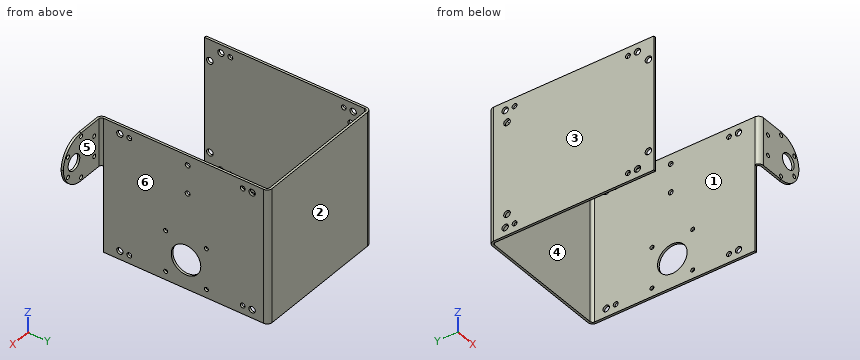
from build123d import *

# Parameters (mm, degrees)
F1_DEPTH  = 101.8535682
F2_R      = 1.5
F2_R_2    = 5.969
F3_DEPTH  = 1.70942
F4_R      = 1.98374
F5_R      = 3.69316
F6_R      = 2.4125047
F6_R_2    = 1.8288
F7_DEPTH  = 105.01884
F8_R      = 11.2530001
F8_R_2    = 1.5
F8_R_3    = 1.8288
F9_DEPTH  = 103.30942
F10_W     = 3.69316
F10_H     = 65.5315682
F11_DEPTH = 40.01516
F12_R     = 18.16099
F13_R     = 2.5
F14_DEPTH = 1.70942


# Not quite as in the source:
# - a fillet or chamfer is up to 0.001 mm smaller than in the source, because OpenCascade refuses the exact size
# - a feature names something its author has since deleted; it is built from what else it names


with BuildPart() as f1:
    # F0 (on Top) → F1 (new body)
    with BuildSketch(Plane.XY):
        Polygon((-1.70942, 0), (0, 0), (0, 123.945777), (101.6, 123.945777), (101.6, -3.69316), (141.61516, -3.69316), (141.61516, -1.98374), (103.30942, -1.98374), (103.30942, 125.655197), (-1.70942, 125.655197), align=None)
    extrude(amount=F1_DEPTH)

    # F2 (on face) → F3 (cut, through all)
    with BuildSketch(Plane.XZ.offset(3.69316)):
        with Locations((136.8723576062, 91.4395682)):
            Circle(F2_R)
        with Locations((130.82016, 83.6925682)):
            Circle(F2_R_2)
        with Locations((136.8723576062, 75.9455682)):
            Circle(F2_R)
        with Locations((123.45416, 99.1865682)):
            Circle(F2_R)
        with Locations((110.0359623938, 91.4395682)):
            Circle(F2_R)
        with Locations((110.0359623938, 75.9455682)):
            Circle(F2_R)
        with Locations((123.45416, 68.1985682)):
            Circle(F2_R)
    extrude(amount=-F3_DEPTH, mode=Mode.SUBTRACT)

    # F4
    f4_edges = [f1.edges().sort_by_distance(p)[0] for p in [
        (0, 123.945777, 50.926784),
        (101.6, 123.945777, 50.926784),
        (103.30942, -1.98374, 50.926784),
    ]]
    fillet(f4_edges, radius=F4_R)

    # F5
    f5_edges = [f1.edges().sort_by_distance(p)[0] for p in [
        (-1.70942, 125.655197, 50.926784),
        (103.30942, 125.655197, 50.926784),
        (101.6, -3.69316, 50.926784),
    ]]
    fillet(f5_edges, radius=F5_R)

    # F6 (on face) → F7 (cut, through all)
    with BuildSketch(Plane(origin=(-1.70942, 0, 0), x_dir=(0, -1, 0), z_dir=(-1, 0, 0))):
        with Locations((-12.5063584, 95.4723182)):
            Circle(F6_R)
        with Locations((-19.6813584, 95.4723182)):
            Circle(F6_R_2)
        with Locations((-105.9738466, 95.4723182)):
            Circle(F6_R_2)
        with Locations((-105.9738466, 6.38125)):
            Circle(F6_R_2)
        with Locations((-19.6813584, 6.38125)):
            Circle(F6_R_2)
        with Locations((-113.1488466, 95.4723182)):
            Circle(F6_R)
        with Locations((-113.1488466, 6.38125)):
            Circle(F6_R)
        with Locations((-12.5063584, 6.38125)):
            Circle(F6_R)
    extrude(amount=-F7_DEPTH, mode=Mode.SUBTRACT)

    # F8 (on face) → F9 (cut, through all)
    with BuildSketch(Plane.YZ.offset(103.30942)):
        with Locations((62.8276025004, 21.8812444)):
            Circle(F8_R)
        with Locations((47.3276081004, 37.3812388)):
            Circle(F8_R_2)
        with Locations((78.3275969004, 37.3812388)):
            Circle(F8_R_2)
        with Locations((78.3275969004, 6.38125)):
            Circle(F8_R_2)
        with Locations((47.3276081004, 6.38125)):
            Circle(F8_R_2)
        with Locations((64.05626, 72.9453964)):
            Circle(F8_R_3)
        with Locations((64.05626, 94.43974)):
            Circle(F8_R_3)
    extrude(amount=-F9_DEPTH, mode=Mode.SUBTRACT)

    # F10 (on face) → F11 (cut, through all)
    with BuildSketch(Plane.YZ.offset(141.61516)):
        with Locations((-1.84658, 32.7657841)):
            Rectangle(F10_W, F10_H)
    extrude(amount=-F11_DEPTH, mode=Mode.SUBTRACT)

    # F12 (radius 18.161 in the source; OpenCascade refuses exactly that, so slightly less here)
    f12_edges = [f1.edges().sort_by_distance(p)[0] for p in [
        (141.61516, -2.83845, 65.531568),
        (141.61516, -2.83845, 101.853568),
    ]]
    fillet(f12_edges, radius=F12_R)

    # F13 (on face) → F14 (cut, through all)
    with BuildSketch(Plane(origin=(-1.70942, 0, 0), x_dir=(0, -1, 0), z_dir=(-1, 0, 0))):
        with Locations((-111.7494286, 16.056229)):
            Circle(F13_R)
        with Locations((-4.0875, 16.056229)):
            Circle(F13_R)
        with Locations((-4.0875, 85.7973392)):
            Circle(F13_R)
        with Locations((-111.7494286, 85.7973392)):
            Circle(F13_R)
    extrude(amount=-F14_DEPTH, mode=Mode.SUBTRACT)


solid = f1.part
Part model, mm, in its own coordinate system. Face numbers are marked on the shaded views. A direction names the side the tool comes from. Coordinates: 2 decimals unless noted, no trailing zeros. Loops run counter-clockwise (first coordinate to the right, second up) from the corner with the lowest first, then second, coordinate; pieces in that order, holes last. Notation, with made-up numbers: (83.25, -8.5) -> (126.25, -8.5) arc R27 cw to (126.25, 23.5) -> close; hole circle Ø4 at (-14, 85). An arc over 180 degrees is marked (long way). Use a Markdown table: item, result. Add a question column.
Item 1: Band-saw the part on B-B on z = 42. Write the cut outline in (x, y).
Item 2: Band-saw the part on A-A on y = 31. Write the cut outline in (x, z), plus the area to 3 significant figures.
Item 3: Band-saw the part on C-C on z = 29. Write the cut outline in (x, y), plus the area to 3 significant figures.
Item 4: Which spindle directions (+Z, -Z, +X, -X, +Y, -Y) get a long thin tool onto all of the face, cutting with end or side? Do the marked faces 1 and 2. Say none if no direction does.
Item 5: Band-saw the part on D-D on x = 116. Write the cut outline in (y, z).
Item 6: Flat gauge pins, fed straight in: P1, Ø5, axis at x = 110.04, z = 75.95, coming from the +Y side; P2, Ø4, axis at y = 4.09, z = 85.8, coming from the +X side; P3, Ø5, axis at x = 60.5, z = 24.5, coming from the -Y side. Where does each tip first touch, or does it go through?
Item 7: Probe probe 1 along X at (y, z) = (4.5, 28); probe 2 along Y at (x, z) = (93.5, 43.5); probe 3 along X at (y, z) = (110, 16). List the from-to ranges inside material, lowest first.
Item 8: Pull direction X, two halves, no side cores. Call the marked faces 3, 4, 5 and 6: +X half, -X half, draft (parallel to the pull), parting line (faces both ways), or undercut.
Geometry says:
| question | item | result |
|---|---|---|
| 1 | outline | (-1.71, 0) -> (0, 0) -> (0, 121.96) arc R1.98 cw to (1.98, 123.95) -> (99.62, 123.95) arc R1.98 cw to (101.6, 121.96) -> (101.6, 0) -> (103.31, 0) -> (103.31, 121.96) arc R3.69 ccw to (99.62, 125.66) -> (1.98, 125.66) arc R3.69 ccw to (-1.71, 121.96) -> close |
| 2 | outline | (-1.71, 0) -> (0, 0) -> (0, 101.85) -> (-1.71, 101.85) -> close; (101.6, 0) -> (103.31, 0) -> (103.31, 101.85) -> (101.6, 101.85) -> close |
| 2 | area | 348 mm² |
| 3 | outline | (-1.71, 0) -> (0, 0) -> (0, 121.96) arc R1.98 cw to (1.98, 123.95) -> (99.62, 123.95) arc R1.98 cw to (101.6, 121.96) -> (101.6, 71.54) -> (103.31, 71.54) -> (103.31, 121.96) arc R3.69 ccw to (99.62, 125.66) -> (1.98, 125.66) arc R3.69 ccw to (-1.71, 121.96) -> close; (101.6, 0) -> (103.31, 0) -> (103.31, 54.11) -> (101.6, 54.11) -> close |
| 3 | area | 569 mm² |
| 4 | face 1 | +Z, -Z, -Y |
| 4 | face 2 | +Z, -Z, +X, -X, +Y |
| 5 | outline | (-3.69, 65.53) -> (-1.98, 65.53) -> (-1.98, 101.85) -> (-3.69, 101.85) -> close |
| 6 | P1 | y = -1.98 |
| 6 | P2 | x = 103.31 |
| 6 | P3 | y = 123.95 |
| 7 | probe 1 | -1.71 to 0, 101.6 to 103.31 |
| 7 | probe 2 | 123.95 to 125.66 |
| 7 | probe 3 | 101.6 to 103.31 |
| 8 | face 3 | -X half |
| 8 | face 4 | undercut |
| 8 | face 5 | draft |
| 8 | face 6 | +X half |
